```python
from build123d import *

# Parameters (mm, degrees)
PAD022_DEPTH    = 10
CHAMFER009_SIZE = 0.5
SKETCH040_R     = 23.9
SKETCH040_R_2   = 22.6
PAD023_DEPTH    = 24
SKETCH041_R     = 23.5
SKETCH041_W     = 20
SKETCH041_H     = 7.75
PAD024_DEPTH    = 24
SKETCH042_R     = 23.9
PAD025_DEPTH    = 4
CHAMFER010_SIZE = 0.5
SKETCH043_R     = 1.5
POCKET013_DEPTH = 15
SKETCH044_R     = 1
POCKET014_DEPTH = 100
SKETCH045_R     = 1.25
POCKET015_DEPTH = 15


with BuildPart() as part:
    # Sketch039 → Pad022 (new body)
    with BuildSketch(Plane.XY):
        with BuildLine():
            ThreePointArc((-14.5, 18.8729965824), (-23.8, 0), (-14.5, -18.8729965824))
            Line((-14.5, -18.8729965824), (14.5, -18.8729965824))
            ThreePointArc((14.5, -18.8729965824), (23.8, 0), (14.5, 18.8729965824))
            Line((-14.5, 18.8729965824), (14.5, 18.8729965824))
        make_face()
        with BuildLine():
            ThreePointArc((-13.8317024681, 17.8729965824), (-22.6, 0), (-13.8317024681, -17.8729965824))
            Line((13.8317024681, -17.8729965824), (-13.8317024681, -17.8729965824))
            ThreePointArc((13.8317024681, -17.8729965824), (22.6, 0), (13.8317024681, 17.8729965824))
            Line((-13.8317024681, 17.8729965824), (13.8317024681, 17.8729965824))
        make_face(mode=Mode.SUBTRACT)
    extrude(amount=PAD022_DEPTH)

    # Chamfer009
    chamfer009_edges = [part.edges().sort_by_distance(p)[0] for p in [
        (0, -18.872997, 10),
        (0, 18.872997, 10),
    ]]
    chamfer(chamfer009_edges, length=CHAMFER009_SIZE)

    # Sketch040 (on Face4 of Chamfer009) → Pad023 (join)
    with BuildSketch(Plane(origin=(0, 0, 0), x_dir=(1, 0, 0), z_dir=(0, 0, -1))):
        Circle(SKETCH040_R)
        Circle(SKETCH040_R_2, mode=Mode.SUBTRACT)
    extrude(amount=PAD023_DEPTH)

    # Sketch041 (on Face4 of Pad023) → Pad024 (join)
    with BuildSketch(Plane.XY):
        Circle(SKETCH041_R)
        with BuildLine():
            Line((-22.4062101037, 2.9532607047), (-17, 2))
            Line((-17, 2), (-17, 1))
            Line((-17, 1), (-19, 1))
            Line((-19, 1), (-19, -1))
            Line((-17, -1), (-19, -1))
            Line((-17, -1), (-17, -2))
            Line((-17, -2), (-22.4062101037, -2.9532607047))
            ThreePointArc((-22.4062101037, -2.9532607047), (-21.7612799705, -6.099729014), (-20.6768211618, -9.1229965824))
            Line((-20.6768211618, -9.1229965824), (20.6768211618, -9.1229965824))
            ThreePointArc((20.6768211618, -9.1229965824), (21.7612799705, -6.099729014), (22.4062101037, -2.9532607047))
            Line((17, -2), (22.4062101037, -2.9532607047))
            Line((17, -1), (17, -2))
            Line((19, -1), (17, -1))
            Line((19, 1), (19, -1))
            Line((19, 1), (17, 1))
            Line((17, 1), (17, 2))
            Line((17, 2), (22.4062101037, 2.9532607047))
            ThreePointArc((22.4062101037, 2.9532607047), (19.5945453266, 11.2611630592), (13.8317024681, 17.8729965824))
            Line((13.8317024681, 17.8729965824), (-13.8317024681, 17.8729965824))
            ThreePointArc((-13.8317024681, 17.8729965824), (-19.5945453266, 11.2611630592), (-22.4062101037, 2.9532607047))
        make_face(mode=Mode.SUBTRACT)
        with Locations((0, -13.9979965824)):
            Rectangle(SKETCH041_W, SKETCH041_H, mode=Mode.SUBTRACT)
    extrude(amount=-PAD024_DEPTH)

    # Sketch042 (on Face49 of Pad024) → Pad025 (join)
    with BuildSketch(Plane(origin=(0, 0, -24), x_dir=(1, 0, 0), z_dir=(0, 0, -1))):
        Circle(SKETCH042_R)
    extrude(amount=PAD025_DEPTH)

    # Chamfer010
    chamfer010_edges = [part.edges().sort_by_distance(p)[0] for p in [
        (-23.9, 0, -28),
    ]]
    chamfer(chamfer010_edges, length=CHAMFER010_SIZE)

    # Sketch043 (on Face4 of Chamfer010) → Pocket013 (cut)
    with BuildSketch(Plane(origin=(0, 0, -28), x_dir=(1, 0, 0), z_dir=(0, 0, -1))):
        with Locations((-16.25, 11.9990624634)):
            Circle(SKETCH043_R)
        with Locations((16.25, 11.9990624634)):
            Circle(SKETCH043_R)
        with Locations((0, -20.2)):
            Circle(SKETCH043_R)
    extrude(amount=-POCKET013_DEPTH, mode=Mode.SUBTRACT)

    # Sketch044 (on Face9 of Pocket013) → Pocket014 (cut)
    with BuildSketch(Plane.XZ.offset(18.8729965824)):
        with Locations((0, 5)):
            Circle(SKETCH044_R)
    extrude(amount=-POCKET014_DEPTH, mode=Mode.SUBTRACT)

    # Sketch045 (on Face29 of Pocket014) → Pocket015 (cut)
    with BuildSketch(Plane.XY):
        with Locations((12.5, -15)):
            Circle(SKETCH045_R)
        with Locations((-12.5, -15)):
            Circle(SKETCH045_R)
    extrude(amount=-POCKET015_DEPTH, mode=Mode.SUBTRACT)


with BuildPart() as part_1:
    # Body017 placement: moved
    add(part.part.moved(Location((0, 0, 200.3))))


solid = part_1.part
```
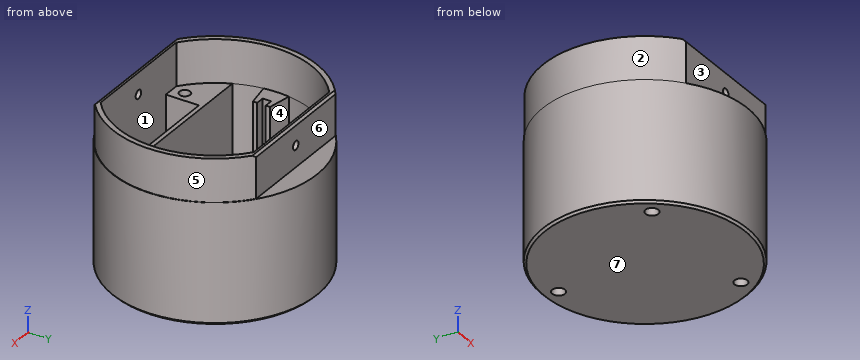
For this review, take the finished solid that the model builds, in its own axes (mm). Face numbers are marked on the shaded views. A direction names the side the tool comes from. Coordinates: 2 decimals unless noted, no trailing zeros. Write each loop counter-clockwise with the first axis right and the second up, starting at its lowest first coordinate (ties: lowest second). Pieces come first, ordered by that corner, then holes. Notation, with made-up numbers: (63, 47.5) -> (113, 47.5) arc R10 ccw to (113, 64.5) -> close; hole circle Ø8 at (74.5, 43). An arc over 180 degrees is marked (long way). Put each result on its own line as item: value.
Q1. Take a section at C-C, the plane z = 196. State the section outline as (x, y) points.
From the geometry:
outline: circle Ø47.8 at (0, 0); hole (-22.41, -2.95) arc R22.6 ccw to (-20.68, -9.12) -> (20.68, -9.12) arc R22.6 ccw to (22.41, -2.95) -> (17, -2) -> (17, -1) -> (19, -1) -> (19, 1) -> (17, 1) -> (17, 2) -> (22.41, 2.95) arc R22.6 ccw to (13.83, 17.87) -> (-13.83, 17.87) arc R22.6 ccw to (-22.41, 2.95) -> (-17, 2) -> (-17, 1) -> (-19, 1) -> (-19, -1) -> (-17, -1) -> (-17, -2) -> close; hole circle Ø2.5 at (-12.5, -15); hole (-10, -17.87) -> (10, -17.87) -> (10, -10.12) -> (-10, -10.12) -> close; hole circle Ø2.5 at (12.5, -15)
Q2. Take a section at B-B, the plane x = 0. Count the separate pieces of the cut face and the enclosed holes in it, then the cut area to 3 significant figures.
From the geometry:
separate pieces: 3
enclosed holes: 0
area: 475 mm2
Q3. Clearance check with flat-ended pins moving along their axes: pin 1 Ø3 at (x, z) = (14.5, 187.5) entering from -Y; pin 2 Ø1 at (x, z) = (-13.5, 198) entering from +Y; pin 3 Ø4 at (y, z) = (14.5, 198.5) entering from -X; pin 4 Ø1.6 at (x, z) = (0, 205.3) entering from -Y. State where each tip first meets the part, or that it passes through.
From the geometry:
pin 1: stops at y = -20.06
pin 2: stops at y = 20.06
pin 3: stops at x = -20.37
pin 4: passes through
Q4. Take a section at A-A, the plane z = 205.3. State the section outline as (x, y) points.
From the geometry:
outline: (-14.5, -18.87) -> (-1, -18.87) -> (-1, -17.87) -> (-13.83, -17.87) arc R22.6 cw to (-13.83, 17.87) -> (-1, 17.87) -> (-1, 18.87) -> (-14.5, 18.87) arc R23.8 ccw to start; (1, -18.87) -> (14.5, -18.87) arc R23.8 ccw to (14.5, 18.87) -> (1, 18.87) -> (1, 17.87) -> (13.83, 17.87) arc R22.6 cw to (13.83, -17.87) -> (1, -17.87) -> close
Q5. Wall thickness on L1, parallel to Y at x = 0, z = 177.25; L2, parallel to Y at x = 4, z = 194; L3, parallel to X at y = -0.5, z = 182: over which ranges is each line inside the solid? List them lowest first.
From the geometry:
L1: y = -23.9 to -17.87, -10.12 to -9.12, 17.87 to 18.7, 21.7 to 23.9
L2: y = -23.56 to -17.87, -10.12 to -9.12, 17.87 to 23.56
L3: x = -23.89 to -19, 19 to 23.89
Q6. The part is to be moulded in two halves that separate along X. For the marked faces 1, 2 and 3, say which applies: +X half, -X half, draft (parallel to the pull), parting line (faces both ways), or undercut.
From the geometry:
face 1: undercut
face 2: -X half
face 3: draft
Q7. Tool access review of the marked faces 4, 5, 6 and 7: name each direction out of +Z, -Z, +X, -X, +Y, -Y from which nothing blocks a thin tool from reaching the whole face with its end or side.
From the geometry:
face 4: +Z
face 5: +Z, +X
face 6: +Z, +X, -X, +Y
face 7: -Z, +X, -X, +Y, -Y
Q8. Take a section at D-D, the plane y = 0. State the section outline as (x, z) points.
From the geometry:
outline: (-23.9, 172.8) -> (-23.4, 172.3) -> (23.4, 172.3) -> (23.9, 172.8) -> (23.9, 200.3) -> (23.8, 200.3) -> (23.8, 210.3) -> (22.6, 210.3) -> (22.6, 200.3) -> (19, 200.3) -> (19, 176.3) -> (-19, 176.3) -> (-19, 200.3) -> (-22.6, 200.3) -> (-22.6, 210.3) -> (-23.8, 210.3) -> (-23.8, 200.3) -> (-23.9, 200.3) -> close
